Geometry: final body of the model. Coordinates: model frame, mm. Give positions to 0.01 mm unless a question says otherwise; leave off trailing zeros. Write each loop counter-clockwise with the first axis right and the second up, starting at its lowest first coordinate (ties: lowest second). Pieces come first, ordered by that corner, then holes. Notation, with made-up numbers: (67.25, -28) -> (114.25, -28) arc R14 cw to (114.25, -24) -> close; hole circle Ø5 at (-19, -16.75). An arc over 180 degrees is marked (long way). Answer in a Markdown table with one row per item. Add a question column.
Item 1: Material intervals for probe 1 along X at (y, z) = (-11, -12.5); probe 2 along Z at (x, y) = (85.25, 68); probe 3 along X at (y, z) = (79, 5), sorted ascending. Write a range as from..to.
Item 2: Section query A-A on y = 63. Output: boundary loops of the cut face in (x, z), plus the area to 3 significant figures.
Item 3: Draft query along Z for faces 1 (the cylindrical face through (65.24, -46.53, 50.24)), 2 (the cylindrical face through (85.082, 72.608, -25.058)), 3 (the flat face through (76.7, 22.42, -32.56)). Return one class per face: +Z half, -Z half, draft (parallel to the pull), parting line (faces both ways), or undercut.
Item 4: First-contact query: P1, Ø5, axis at y = 66.5, z = -18, coming from the +X side; P2, Ø4, axis at y = -21.5, z = 23, coming from the +X side; P3, Ø1.5, axis at y = 28, z = 5, coming from the +X side. Flat tips, straight axial feed; report the tip coordinate or a pass-through.
Item 5: Section query B-B on z = -19.5. Output: boundary loops of the cut face in (x, y).
```python
from build123d import *

# Parameters (mm, degrees)
BOSS_EXTRUDE2_START = 10
SKETCH5_R           = 3.875
SKETCH5_R_2         = 4
BOSS_EXTRUDE2_DEPTH = 4
FILLET1_R           = 3
FILLET2_R           = 3


with BuildPart() as part:
    # Sketch5 → Boss-Extrude2 (new body)
    with BuildSketch(Plane(origin=(59.169020247, -9.881108749, 0), x_dir=(0, 0, -1), z_dir=(0.9863408748405357, -0.16471696518211734, 0)).offset(BOSS_EXTRUDE2_START)):
        Polygon((-51.1, 106.13567165), (65.395465612, 106.13567165), (0, -36.047454034), (-51.1, -36.047454034), align=None)
        with Locations(Location((-31.1, 86.13567165, 0), (0, 0, 90))):
            Circle(SKETCH5_R, mode=Mode.SUBTRACT)
        with Locations(Location((28.9, 86.13567165, 0), (0, 0, 90))):
            Circle(SKETCH5_R, mode=Mode.SUBTRACT)
        with Locations(Location((-8.6, 41.13567165, 0), (0, 0, 90))):
            Circle(SKETCH5_R_2, mode=Mode.SUBTRACT)
        with Locations(Location((-21.1, -16.047454034, 0), (0, 0, 90))):
            Circle(SKETCH5_R, mode=Mode.SUBTRACT)
    extrude(amount=BOSS_EXTRUDE2_DEPTH)

    # Fillet1
    fillet1_edges = [part.edges().sort_by_distance(p)[0] for p in [
        (65.067483514, -47.412789679, 0),
        (65.067483514, -47.412789679, 51.1),
    ]]
    fillet(fillet1_edges, radius=FILLET1_R)

    # Fillet2
    fillet2_edges = [part.edges().sort_by_distance(p)[0] for p in [
        (88.487456476, 92.828238896, 51.1),
        (88.487456476, 92.828238896, -65.395465612),
    ]]
    fillet(fillet2_edges, radius=FILLET2_R)


solid = part.part
```
Findings below:
| question | item | result |
|---|---|---|
| 1 | probe 1 | x = 69.12..73.18 |
| 1 | probe 2 | z = -53.89..51.1 |
| 1 | probe 3 | x = 84.15..88.21 |
| 2 | outline | (81.48, -51.33) -> (85.53, -51.64) -> (85.53, 51.1) -> (81.48, 51.1) -> close |
| 2 | area | 416 mm^2 |
| 3 | face 1 | +Z half |
| 3 | face 2 | undercut |
| 3 | face 3 | -Z half |
| 4 | P1 | stops at x = 86.54 |
| 4 | P2 | stops at x = 71.76 |
| 4 | P3 | stops at x = 79.8 |
| 5 | outline | (70.08, -5.27) -> (74.02, -5.92) -> (90.46, 92.5) -> (86.51, 93.16) -> close |
